Source: CAD feature listing. Evaluate the final solid. Frame: model axes, mm. Coordinates: 2 decimals unless noted, no trailing zeros. Write each loop counter-clockwise with the first axis right and the second up, starting at its lowest first coordinate (ties: lowest second). Pieces come first, ordered by that corner, then holes. Notation, with made-up numbers: (53.5, 84.25) - (103.5, 84.25) arc R27 ccw to (103.5, 100.25) - close; hole circle Ø3 at (-37, 44). An arc over 180 degrees is marked (long way). One line per item, written item: value.
from build123d import *

# Parameters (mm, degrees)
SKETCH_6_R          = 15
CUT_EXTRUDE_1_DEPTH = 5
CHAMFER_1_SIZE      = 1
CHAMFER_1_SIZE2     = 1.5


with BuildPart() as part:
    # Эскиз5 → Повернуть1 (revolve)
    with BuildSketch(Plane(origin=(0, 0, 0), x_dir=(0, 0, -1), z_dir=(1, 0, 0))):
        with BuildLine():
            Line((-4, 0), (-4, 15))
            Line((-4, 15), (-2.303039929, 15))
            ThreePointArc((-2.303039929, 15), (-0.579113709, 7.587884964), (0, 0))
            Line((0, 0), (-4, 0))
        make_face()
    revolve(axis=Axis((0, 0, -1), (0, 0, 1)))

    # Эскиз6 → Вырез-Вытянуть1 (cut, through all)
    with BuildSketch(Plane.XY.offset(4)):
        Circle(SKETCH_6_R)
        with BuildLine():
            Line((-3, -14), (-3, 14))
            ThreePointArc((-3, 14), (11, 0), (-3, -14))
        make_face(mode=Mode.SUBTRACT)
    extrude(amount=-CUT_EXTRUDE_1_DEPTH, mode=Mode.SUBTRACT)

    # Фаска1
    chamfer_1_edges = [part.edges().sort_by_distance(p)[0] for p in [
        (-3, 0, 4),
    ]]
    chamfer_1_side = [part.faces().sort_by_distance(p)[0] for p in [
        (-3, 0, 2.321648578),
    ]]
    chamfer(chamfer_1_edges, length=CHAMFER_1_SIZE, length2=CHAMFER_1_SIZE2, reference=chamfer_1_side[0])


solid = part.part
1) Section query A-A on y = 0. Output: boundary loops of the cut face in (x, z) (3 decimals).
Values found:
outline: (-3, 0.09) arc R50 ccw to (11, 1.225) - (11, 4) - (-1.5, 4) - (-3, 3) - close
2) Section query C-C on y = -3. Output: boundary loops of the cut face in (x, z), then the cut area to 3 significant figures.
Values found:
outline: (-3, 0.18) arc R49.91 ccw to (10.67, 1.25) - (10.67, 4) - (-1.5, 4) - (-3, 3) - close
area: 48.5 mm2
3) Material intervals for line 1 (X direction, y = 6.25, z = 2.1); line 2 (Y direction, x = 4.5, z = 3.5); line 3 (Y direction, x = 2, z = 2.7), sorted ascending.
Values found:
line 1: -3 to 9.53
line 2: -11.82 to 11.82
line 3: -13.08 to 13.08
4) Section query B-B on z = 0.75. Output: boundary loops of the cut face in (x, y), then the cut area to 3 significant figures.
Values found:
outline: (-3, -8.09) arc R8.63 ccw (long way) to (-3, 8.09) - close
area: 168 mm2
5) Contact query for flat-ended pins moving along their axis: P1, Ø1, axis at x = 3, y = 5.5, coming from the -Z side; P2, Ø1.5, axis at x = 4.5, z = 1, coming from the -Y side; P3, Ø5, axis at x = 7.5, y = -9.5, coming from the -Z side. Output: stop coordinate, or through.
Values found:
P1: z = 0.33
P2: y = -12.05
P3: z = 0.93
